from build123d import *

# Parameters (mm, degrees)
SKETCH1_R           = 2
SKETCH1_R_2         = 1.5
BOSS_EXTRUDE1_DEPTH = 5
SKETCH2_W           = 4
SKETCH2_H           = 16
CUT_EXTRUDE1_DEPTH  = 5
BOSS_EXTRUDE3_DEPTH = 25
SKETCH4_W           = 72
SKETCH4_H           = 54
BOSS_EXTRUDE4_DEPTH = 5
SKETCH5_W           = 40
SKETCH5_H           = 20
CUT_EXTRUDE2_DEPTH  = 123.576506721
SKETCH6_W           = 20
SKETCH6_H           = 6
CUT_EXTRUDE4_DEPTH  = 10
BOSS_EXTRUDE5_START = -5
SKETCH7_R           = 4
BOSS_EXTRUDE5_DEPTH = 5
SKETCH8_R           = 2
CUT_EXTRUDE5_DEPTH  = 10
CUT_EXTRUDE6_START  = 10
SKETCH9_R           = 4
CUT_EXTRUDE6_DEPTH  = 10
BOSS_EXTRUDE6_START = 5
SKETCH10_R          = 6
BOSS_EXTRUDE6_DEPTH = 30
SKETCH11_R          = 2
CUT_EXTRUDE7_DEPTH  = 10
CUT_EXTRUDE8_START  = 20
SKETCH12_R          = 4.5
CUT_EXTRUDE8_DEPTH  = 129.434311913
SKETCH14_R          = 4.5
CUT_EXTRUDE11_DEPTH = 108.158760724
SKETCH13_R          = 1.5
BOSS_EXTRUDE8_DEPTH = 3
CHAMFER2_SIZE       = 1
CHAMFER3_SIZE       = 2
CHAMFER4_SIZE       = 2
CHAMFER5_SIZE       = 2
CUT_EXTRUDE15_START = -3
SKETCH13_3_R        = 1.5
CUT_EXTRUDE15_DEPTH = 3
CUT_EXTRUDE18_START = 3
SKETCH13_5_R        = 1.5
CUT_EXTRUDE18_DEPTH = 6
SKETCH23_R          = 1.5
CUT_EXTRUDE19_DEPTH = 6


with BuildPart() as part:
    # Sketch1 → Boss-Extrude1 (new body)
    with BuildSketch(Plane(origin=(0, 0, 0), x_dir=(1, 0, 0), z_dir=(0, 1, 0))):
        Polygon((0, 34), (0, -34), (13, -47), (32, -47), (32, -34), (55, -34), (55, -47), (61, -47), (63, -45), (93, -45), (93, -41), (75, -41), (75, -37), (93, -37), (93, -22), (33, -22), (21, -10), (21, 10), (33, 22), (93, 22), (93, 37), (75, 37), (75, 41), (93, 41), (93, 45), (63, 45), (61, 47), (55, 47), (55, 34), (32, 34), (32, 47), (13, 47), align=None)
        with Locations(Location((13, -10, 0), (0, 0, 270))):
            Circle(SKETCH1_R, mode=Mode.SUBTRACT)
        with Locations(Location((29, -40, 0), (0, 0, 270))):
            Circle(SKETCH1_R_2, mode=Mode.SUBTRACT)
        with Locations(Location((58, -40, 0), (0, 0, 270))):
            Circle(SKETCH1_R_2, mode=Mode.SUBTRACT)
        with Locations(Location((63, -27, 0), (0, 0, 270))):
            Circle(SKETCH1_R, mode=Mode.SUBTRACT)
        with Locations(Location((13, 10, 0), (0, 0, 90))):
            Circle(SKETCH1_R, mode=Mode.SUBTRACT)
        with Locations(Location((29, 40, 0), (0, 0, 90))):
            Circle(SKETCH1_R_2, mode=Mode.SUBTRACT)
        with Locations(Location((58, 40, 0), (0, 0, 90))):
            Circle(SKETCH1_R_2, mode=Mode.SUBTRACT)
        with Locations(Location((63, 27, 0), (0, 0, 90))):
            Circle(SKETCH1_R, mode=Mode.SUBTRACT)
    extrude(amount=BOSS_EXTRUDE1_DEPTH)

    # Sketch2 → Cut-Extrude1 (cut)
    with BuildSketch(Plane(origin=(0, 5, 0), x_dir=(1, 0, 0), z_dir=(0, 1, 0))):
        Polygon((17, 33.205766921), (17, 36.408329997), (4, 26), (4, 12), (8, 12), (8, 26), align=None)
        with Locations((6, 0)):
            Rectangle(SKETCH2_W, SKETCH2_H)
        Polygon((17, -33.205766921), (17, -36.408329997), (4, -26), (4, -12), (8, -12), (8, -26), align=None)
    extrude(amount=-CUT_EXTRUDE1_DEPTH, mode=Mode.SUBTRACT)

    # Sketch3 → Boss-Extrude3 (add)
    with BuildSketch(Plane(origin=(0, 5, 0), x_dir=(1, 0, 0), z_dir=(0, 1, 0))):
        Polygon((21, 27), (21, 10), (33, 22), (93, 22), (93, 27), align=None)
        Polygon((93, -27), (93, -22), (33, -22), (21, -10), (21, -27), align=None)
    extrude(amount=BOSS_EXTRUDE3_DEPTH)

    # Sketch4 → Boss-Extrude4 (add)
    with BuildSketch(Plane(origin=(0, 30, 0), x_dir=(1, 0, 0), z_dir=(0, 1, 0))):
        with Locations((57, 0)):
            Rectangle(SKETCH4_W, SKETCH4_H)
    extrude(amount=-BOSS_EXTRUDE4_DEPTH)

    # Sketch5 → Cut-Extrude2 (cut, through all)
    with BuildSketch(Plane.XY.offset(27)):
        with Locations((53, 15)):
            Rectangle(SKETCH5_W, SKETCH5_H)
    extrude(amount=-CUT_EXTRUDE2_DEPTH, mode=Mode.SUBTRACT)

    # Sketch6 → Cut-Extrude4 (cut)
    with BuildSketch(Plane(origin=(0, 30, 0), x_dir=(1, 0, 0), z_dir=(0, 1, 0))):
        with Locations((63, 24)):
            Rectangle(SKETCH6_W, SKETCH6_H)
        with Locations((63, -24)):
            Rectangle(SKETCH6_W, SKETCH6_H)
    extrude(amount=-CUT_EXTRUDE4_DEPTH, mode=Mode.SUBTRACT)

    # Sketch7 → Boss-Extrude5 (add)
    with BuildSketch(Plane.XZ.offset(-25).offset(BOSS_EXTRUDE5_START)):
        with Locations(Location((83, 21, 0), (0, 0, 270))):
            Circle(SKETCH7_R)
        with Locations(Location((83, -21, 0), (0, 0, 270))):
            Circle(SKETCH7_R)
    extrude(amount=-BOSS_EXTRUDE5_DEPTH)

    # Sketch8 → Cut-Extrude5 (cut)
    with BuildSketch(Plane(origin=(0, 35, 0), x_dir=(1, 0, 0), z_dir=(0, 1, 0))):
        with Locations(Location((83, 21, 0), (0, 0, 270))):
            Circle(SKETCH8_R)
    cut_extrude5 = extrude(amount=-CUT_EXTRUDE5_DEPTH, mode=Mode.SUBTRACT)

    # Sketch9 → Cut-Extrude6 (cut)
    with BuildSketch(Plane.XZ.offset(-25).offset(CUT_EXTRUDE6_START)):
        with Locations(Location((83, -21, 0), (0, 0, 270))):
            Circle(SKETCH9_R)
    cut_extrude6 = extrude(amount=-CUT_EXTRUDE6_DEPTH, mode=Mode.SUBTRACT)

    # Sketch10 → Boss-Extrude6 (add)
    with BuildSketch(Plane(origin=(0, 30, 0), x_dir=(1, 0, 0), z_dir=(0, 1, 0)).offset(BOSS_EXTRUDE6_START)):
        with Locations(Location((21, 21, 0), (0, 0, 270))):
            Circle(SKETCH10_R)
    boss_extrude6 = extrude(amount=-BOSS_EXTRUDE6_DEPTH)

    # Sketch11 → Cut-Extrude7 (cut)
    with BuildSketch(Plane(origin=(0, 35, 0), x_dir=(1, 0, 0), z_dir=(0, 1, 0))):
        with Locations(Location((21, 21, 0), (0, 0, 270))):
            Circle(SKETCH11_R)
    cut_extrude7 = extrude(amount=-CUT_EXTRUDE7_DEPTH, mode=Mode.SUBTRACT)

    # Sketch12 → Cut-Extrude8 (cut, through all)
    with BuildSketch(Plane(origin=(0, 5, 0), x_dir=(1, 0, 0), z_dir=(0, 1, 0)).offset(CUT_EXTRUDE8_START)):
        with Locations(Location((21, 21, 0), (0, 0, 270))):
            Circle(SKETCH12_R)
    extrude(amount=-CUT_EXTRUDE8_DEPTH, mode=Mode.SUBTRACT)

    # Mirror11: Cut-Extrude5, Cut-Extrude6 across plane
    add(cut_extrude5.mirror(Plane.XY), mode=Mode.SUBTRACT)
    add(cut_extrude6.mirror(Plane.XY), mode=Mode.SUBTRACT)

    # Mirror12: Boss-Extrude6 across plane
    add(boss_extrude6.mirror(Plane.XY))

    # Mirror16: Cut-Extrude7 across plane
    add(cut_extrude7.mirror(Plane.XY), mode=Mode.SUBTRACT)

    # Sketch14 → Cut-Extrude11 (cut, through all)
    with BuildSketch(Plane(origin=(0, 25, 0), x_dir=(1, 0, 0), z_dir=(0, 1, 0))):
        with Locations(Location((21, -21, 0), (0, 0, 270))):
            Circle(SKETCH14_R)
    extrude(amount=-CUT_EXTRUDE11_DEPTH, mode=Mode.SUBTRACT)

    # Sketch13 → Boss-Extrude8 (add)
    with BuildSketch(Plane(origin=(93, 0, 0), x_dir=(0, 0, -1), z_dir=(1, 0, 0))):
        with Locations(Location((24.5, 5, 0), (0, 0, 180))):
            Circle(SKETCH13_R)
    boss_extrude8 = extrude(amount=BOSS_EXTRUDE8_DEPTH)

    # Mirror19: Boss-Extrude8 across plane
    add(boss_extrude8.mirror(Plane.XY))

    # Chamfer2
    chamfer2_edges = [part.edges().sort_by_distance(p)[0] for p in [
        (83, 35, 25),
        (83, 35, -17),
    ]]
    chamfer(chamfer2_edges, length=CHAMFER2_SIZE)

    # Chamfer3
    chamfer3_edges = [part.edges().sort_by_distance(p)[0] for p in [
        (22.5, 5, -47),
        (6.5, 5, -40.5),
        (0, 5, 0),
        (6.5, 5, 40.5),
        (21, 35, -27),
        (21, 35, 27),
        (22.5, 5, 47),
    ]]
    chamfer(chamfer3_edges, length=CHAMFER3_SIZE)

    # Chamfer4
    chamfer4_edges = [part.edges().sort_by_distance(p)[0] for p in [
        (83, 5, -27),
        (83, 5, 27),
        (73, 5, 24.5),
        (73, 5, -24.5),
    ]]
    chamfer(chamfer4_edges, length=CHAMFER4_SIZE)

    # Chamfer5
    chamfer5_edges = [part.edges().sort_by_distance(p)[0] for p in [
        (83, 25, -23),
        (83, 25, 23),
    ]]
    chamfer(chamfer5_edges, length=CHAMFER5_SIZE - 0.0001)  # a hair under: the kernel refuses the full size

    # Sketch13<3> → Cut-Extrude15 (cut)
    with BuildSketch(Plane(origin=(93, 0, 0), x_dir=(0, 0, -1), z_dir=(1, 0, 0)).offset(CUT_EXTRUDE15_START)):
        with Locations((24.5, 5)):
            Circle(SKETCH13_3_R)
    extrude(amount=CUT_EXTRUDE15_DEPTH, mode=Mode.SUBTRACT)


with BuildPart() as cut_extrude15_piece_1:
    # of the separate pieces the step leaves, piece 1, a body of its own (cut_extrude15_pieces)
    add(part.part.solids().sort_by_distance((83, 25, -17.0001))[0])

    # Sketch23 → Cut-Extrude19 (cut)
    with BuildSketch(Plane(origin=(96, 0, 0), x_dir=(0, 0, -1), z_dir=(1, 0, 0))):
        with Locations((-24.5, 5)):
            Circle(SKETCH23_R)
    extrude(amount=-CUT_EXTRUDE19_DEPTH, mode=Mode.SUBTRACT)


with BuildPart() as cut_extrude15_piece_2:
    # of the separate pieces the step leaves, piece 2, a body of its own (cut_extrude15_pieces)
    add(part.part.solids().sort_by_distance((96, 5, -23))[0])

    # Sketch13<5> → Cut-Extrude18 (cut)
    with BuildSketch(Plane(origin=(93, 0, 0), x_dir=(0, 0, -1), z_dir=(1, 0, 0)).offset(CUT_EXTRUDE18_START)):
        with Locations((24.5, 5)):
            Circle(SKETCH13_5_R)
    extrude(amount=-CUT_EXTRUDE18_DEPTH, mode=Mode.SUBTRACT)


solid = cut_extrude15_piece_1.part
CAD build for the part. Positions are in the model's coordinates, mm. A direction names the side the tool comes from. Coordinates: 2 decimals unless noted, no trailing zeros. Write each loop counter-clockwise with the first axis right and the second up, starting at its lowest first coordinate (ties: lowest second). Pieces come first, ordered by that corner, then holes. Notation, with made-up numbers: M 38,20.5 L 55,20.5 A17 ccw 55,52.5 Z; hole C 17,25.5 d9. An arc over 180 degrees is marked long. Answer as a JSON object with one key per item and string values. Group by question number.
1) Saw through at B-B (x = 58). Write the cut outline in (y, z), plus the area to 3 significant figures.
2) Tool access for faces 5 (the face through (43, 2, 34)), 6 (the face through (84, 2, 37)), 7 (the face through (8, 3, -19)), 8 (the face through (21, 2, 0)): list every direction of +Z, -Z, +X, -X, +Y, -Y with a clear straight run to the whole face (end or side of a thin tool).
3) Saw through at A-A (y = 12). Write the cut outline in (x, z).
4) Pin check, flat tips, straight feed: pin 1 Ø1.5 at (x, z) = (33.5, 1.5) entering from +Y; pin 2 Ø12 at (x, y) = (16.5, 25.5) entering from +Z; pin 3 Ø3 at (y, z) = (19.5, -23.5) entering from -X. Stop position of each tip, or through.
5) Saw through at D-D (z = -3). Write the cut outline in (x, y).
6) Wall check: line 1 (X direction, y = 31.5, z = -21); line 2 (X direction, y = 15.5, z = -21); line 3 (Z direction, x = 32, y = 17.5). Give the ranges that are in metal, low to high. Write a range as from..to.
7) Mould opens along Z. For faces 1 (the face through (84, 2, -41)), 2 (the face through (73, 18, 24)), 3 (the face through (6, 1, 40)), 4 (the face through (85, 31, -21)) say: +Z half, -Z half, draft (parallel to the pull), parting line (faces both ways), or undercut.
8) Saw through at C-C (x = 36.5). Write the cut outline in (y, z).
Values follow:
{
 "1": {"outline": "M 0,-47 L 5,-47 L 5,-41.5 L 0,-41.5 Z; M 0,-38.5 L 5,-38.5 L 5,-22 L 0,-22 Z; M 0,22 L 5,22 L 5,38.5 L 0,38.5 Z; M 0,41.5 L 5,41.5 L 5,47 L 0,47 Z; M 25,-21 L 30,-21 L 30,21 L 25,21 Z", "area": "430 mm2"},
 "2": {"face 5": "+Z, +Y, -Y", "face 6": "+X, +Y, -Y", "face 7": "+Y, -Y", "face 8": "+X, -Y"},
 "3": {"outline": "M 21,-27 L 33,-27 L 33,-22 L 21,-10 L 21,-15 A6 ccw Z; M 21,10 L 33,22 L 33,27 L 21,27 A6 ccw 21,15 Z; M 73,-27 L 93,-27 L 93,-22 L 73,-22 Z; M 73,22 L 93,22 L 93,27 L 73,27 Z; hole C 21,-21 d9; hole C 21,21 d9"},
 "4": {"pin 1": "stops at y = 30", "pin 2": "stops at z = 27", "pin 3": "stops at x = 15.08"},
 "5": {"outline": "M 0,0 L 4,0 L 4,5 L 2,5 L 0,3 Z; M 8,0 L 21,0 L 21,5 L 8,5 Z; M 21,25 L 93,25 L 93,30 L 21,30 Z"},
 "6": {"line 1": "x = 15..19, 23..27, 79..81, 85..87", "line 2": "x = 15..16.5, 25.5..32", "line 3": "z = -27..-21, 21..27"},
 "7": {"face 1": "undercut", "face 2": "draft", "face 3": "+Z half", "face 4": "undercut"},
 "8": {"outline": "M 0,-34 L 5,-34 L 5,-22 L 0,-22 Z; M 0,22 L 5,22 L 5,34 L 0,34 Z; M 25,-27 L 30,-27 L 30,27 L 25,27 Z"}
}
